Geometry: final body of the model. Coordinates: model frame, mm. A direction names the side the tool comes from. Give positions to 0.01 mm unless a question says otherwise; leave off trailing zeros. Loops run counter-clockwise (first coordinate to the right, second up) from the corner with the lowest first, then second, coordinate; pieces in that order, holes last. Notation, with made-up numbers: M 0,-24.5 L 50,-24.5 A29 ccw 50,14.5 Z; hole C 41.25,-14 d5. An arc over 180 degrees is marked long. Put each result on its own line as item: value.
```python
from build123d import *

# Parameters (mm, degrees)
PAD_DEPTH       = 3
SKETCH005_R     = 1.75
POCKET004_DEPTH = 3.001
SKETCH006_W     = 15
SKETCH006_H     = 44
POCKET_DEPTH    = 3.001
FILLET_R        = 2


with BuildPart() as part:
    # Sketch → Pad (new body)
    with BuildSketch(Plane.XY):
        Polygon((-61, 71), (-54, 78), (54, 78), (61, 71), (61, -71), (54, -78), (-54, -78), (-61, -71), align=None)
    extrude(amount=PAD_DEPTH)

    # Sketch005 → Pocket004 (cut, through all)
    with BuildSketch(Plane.XY.offset(3)):
        with Locations((-54, 71)):
            Circle(SKETCH005_R)
        with Locations((54, 71)):
            Circle(SKETCH005_R)
        with Locations((-54, -71)):
            Circle(SKETCH005_R)
        with Locations((54, -71)):
            Circle(SKETCH005_R)
    extrude(amount=-POCKET004_DEPTH, mode=Mode.SUBTRACT)

    # Sketch006 (on Face5 of Pocket004) → Pocket (cut, through all)
    with BuildSketch(Plane.XY.offset(3)):
        with Locations((-53.5, -2.7)):
            Rectangle(SKETCH006_W, SKETCH006_H)
    extrude(amount=-POCKET_DEPTH, mode=Mode.SUBTRACT)

    # Fillet
    fillet_edges = [part.edges().sort_by_distance(p)[0] for p in [
        (-46, 19.3, 1.5),
        (-46, -24.7, 1.5),
    ]]
    fillet(fillet_edges, radius=FILLET_R)


solid = part.part
```
Item 1: Section B-B on y = -13. Output: boundary loops of the cut face in (x, z), then the cut area to 3 significant figures.
Output values:
outline: M -46,0 L 61,0 L 61,3 L -46,3 Z
area: 321 mm²
Item 2: Pin query (flat end, axial travel): pin 1 Ø2 at (x, y) = (-54, -71) entering from +Z. Return the tip coordinate at first contact, or that it passes through.
Output values:
pin 1: through
Item 3: Mould query, pull axis X, two halves, no side actions, for faces 1 (the flat face through (57, 75, 1)), 2 (the flat face through (-57, -75, 1)), 3 (the flat face through (-1, 78, 1)), 4 (the cylindrical face through (55.617, -71.67, 1.521)). Classes: pulls with the +X half, pulls with the -X half, needs draft (parallel to the pull), parting line crosses it, or undercut.
Output values:
face 1: pulls with the +X half
face 2: pulls with the -X half
face 3: needs draft
face 4: undercut
Item 4: Set-up query: faces 5 (the flat face through (1, 1, 3)), 6 (the flat face through (-55, -24.7, 2)). Return all of +Z, -Z, +X, -X, +Y, -Y with unobstructed straight access to the full face (end or side cutting, diameter ignored); none if empty.
Output values:
face 5: +Z, +X, -X, +Y, -Y
face 6: +Z, -Z, -X
Item 5: Section A-A on z = 2. Output: boundary loops of the cut face in (x, y).
Output values:
outline: M -61,-71 L -54,-78 L 54,-78 L 61,-71 L 61,71 L 54,78 L -54,78 L -61,71 L -61,19.3 L -48,19.3 A2 cw -46,17.3 L -46,-22.7 A2 cw -48,-24.7 L -61,-24.7 Z; hole C -54,-71 d3.5; hole C -54,71 d3.5; hole C 54,-71 d3.5; hole C 54,71 d3.5
Item 6: Line query: probe 1 along Y at (x, z) = (54, 1.8); probe 2 along X at (y, z) = (-71, 1.65); probe 3 along Y at (x, z) = (-54, 1.7). Output: solid intervals per line, ascending. Write a range as [from, to].
Output values:
probe 1: [-78, -72.75], [-69.25, 69.25], [72.75, 78]
probe 2: [-61, -55.75], [-52.25, 52.25], [55.75, 61]
probe 3: [-78, -72.75], [-69.25, -24.7], [19.3, 69.25], [72.75, 78]
